```python
from build123d import *

# Parameters (mm, degrees)
SKETCH1_R           = 1.625
BOSS_EXTRUDE1_DEPTH = 2.5
FILLET1_R           = 5
SKETCH3_R           = 4.125
CUT_EXTRUDE2_DEPTH  = 71.75485849
CUT_EXTRUDE3_DEPTH  = 71.75485849
FILLET2_R           = 10
CHAMFER1_SIZE       = 1


with BuildPart() as part:
    # Sketch1 → Boss-Extrude1 (new body)
    with BuildSketch(Plane(origin=(0, 0, 0), x_dir=(1, 0, 0), z_dir=(0, 1, 0))):
        with BuildLine():
            ThreePointArc((50, 0), (-27.838821814, 41.533119315), (-19, -46.249324319))
            Line((-19, -46.249324319), (-19, -11))
            Line((-19, -11), (19, -11))
            Line((19, -11), (19, -46.249324319))
            ThreePointArc((19, -46.249324319), (41.533119315, -27.838821814), (50, 0))
        make_face()
        with Locations(Location((-15, 5, 0), (0, 0, 270))):
            Circle(SKETCH1_R, mode=Mode.SUBTRACT)
        with Locations(Location((15, 5, 0), (0, 0, 270))):
            Circle(SKETCH1_R, mode=Mode.SUBTRACT)
    extrude(amount=BOSS_EXTRUDE1_DEPTH)

    # Fillet1
    fillet1_edges = [part.edges().sort_by_distance(p)[0] for p in [
        (19, 1.25, 46.249324319),
        (19, 1.25, 11),
        (-19, 1.25, 11),
        (-19, 1.25, 46.249324319),
    ]]
    fillet(fillet1_edges, radius=FILLET1_R)

    # Sketch3 → Cut-Extrude2 (cut, through all)
    with BuildSketch(Plane(origin=(0, 2.5, 0), x_dir=(1, 0, 0), z_dir=(0, 1, 0))):
        with Locations(Location((0, 33.5, 0), (0, 0, 270))):
            Circle(SKETCH3_R)
        with Locations(Location((29.011851027, -16.75, 0), (0, 0, 270))):
            Circle(SKETCH3_R)
        with Locations(Location((-29.011851027, -16.75, 0), (0, 0, 270))):
            Circle(SKETCH3_R)
    extrude(amount=-CUT_EXTRUDE2_DEPTH, mode=Mode.SUBTRACT)

    # Sketch4 → Cut-Extrude3 (cut, through all)
    with BuildSketch(Plane(origin=(0, 2.5, 0), x_dir=(1, 0, 0), z_dir=(0, 1, 0))):
        with BuildLine():
            ThreePointArc((-19, -30.369481935), (-30.236455629, -33.609056698), (-40.88679997, -28.779673178))
            ThreePointArc((-40.88679997, -28.779673178), (-34.446124239, -36.241751129), (-26.666666667, -42.295258468))
            ThreePointArc((-26.666666667, -42.295258468), (-21.584770542, -42.4437078), (-19, -38.065732621))
            Line((-19, -38.065732621), (-19, -30.369481935))
        make_face()
        with BuildLine():
            Line((19, -30.369481935), (19, -38.065732621))
            ThreePointArc((19, -38.065732621), (21.584770542, -42.4437078), (26.666666667, -42.295258468))
            ThreePointArc((26.666666667, -42.295258468), (34.446124239, -36.241751129), (40.88679997, -28.779673178))
            ThreePointArc((40.88679997, -28.779673178), (30.236455629, -33.609056698), (19, -30.369481935))
        make_face()
        with BuildLine():
            ThreePointArc((-6.8e-08, 50), (-42.136436408, 26.916922685), (-45.36732807, -21.019170864))
            ThreePointArc((-45.36732807, -21.019170864), (-44.746417351, -10.573360804), (-38.095485584, -2.49464899))
            Line((-38.095485584, -2.49464899), (-20.59178284, 8.658863751))
            Line((-20.59178284, 8.658863751), (-16.301275801, 36.053117163))
            ThreePointArc((-16.301275801, 36.053117163), (-10.7266856, 46.037472474), (-6.8e-08, 50))
        make_face()
        with BuildLine():
            ThreePointArc((45.36732807, -21.019170864), (42.136436371, 26.916922743), (-6.8e-08, 50))
            ThreePointArc((-6.8e-08, 50), (10.726685548, 46.037472518), (16.301275801, 36.053117163))
            Line((16.301275801, 36.053117163), (20.59178284, 8.658863751))
            Line((20.59178284, 8.658863751), (38.095485584, -2.49464899))
            ThreePointArc((38.095485584, -2.49464899), (44.746417351, -10.573360804), (45.36732807, -21.019170864))
        make_face()
    extrude(amount=-CUT_EXTRUDE3_DEPTH, mode=Mode.SUBTRACT)

    # Fillet2
    fillet2_edges = [part.edges().sort_by_distance(p)[0] for p in [
        (40.88679997, 1.25, 28.779673178),
        (-45.36732807, 1.25, 21.019170864),
        (-20.59178284, 1.25, -8.658863751),
        (45.36732807, 1.25, 21.019170864),
        (20.59178284, 1.25, -8.658863751),
        (-40.88679997, 1.25, 28.779673178),
        (-19, 1.25, 30.369481935),
        (19, 1.25, 30.369481935),
    ]]
    fillet(fillet2_edges, radius=FILLET2_R)

    # Chamfer1
    chamfer1_edges = [part.edges().sort_by_distance(p)[0] for p in [
        (-44.388404549, 2.5, 9.729383862),
        (-18.097260259, 2.5, -24.5860218),
        (-44.388404549, 0, 9.729383862),
        (-18.097260259, 0, -24.5860218),
        (-43.301270189, 2.5, 25),
        (-43.301270189, 0, 25),
        (-34.559008869, 2.5, 32.717356984),
        (-19, 2.5, 19.826732149),
        (34.559008869, 2.5, 32.717356984),
        (43.301270189, 2.5, 25),
        (44.388404549, 2.5, 9.729383862),
        (31.247232254, 2.5, -1.86911803),
        (-31.247232254, 2.5, -1.86911803),
        (21.922865426, 2.5, 30.718460138),
        (-21.922865426, 2.5, 30.718460138),
        (40.660570606, 2.5, 28.929698969),
        (45.384139534, 2.5, 20.748237593),
        (-45.384139534, 2.5, 20.748237593),
        (-40.660570606, 2.5, 28.929698969),
        (-34.559008869, 0, 32.717356984),
        (-31.247232254, 0, -1.86911803),
        (31.247232254, 0, -1.86911803),
        (44.388404549, 0, 9.729383862),
        (43.301270189, 0, 25),
        (34.559008869, 0, 32.717356984),
        (-19, 0, 19.826732149),
        (21.922865426, 0, 30.718460138),
        (-21.922865426, 0, 30.718460138),
        (40.660570606, 0, 28.929698969),
        (45.384139534, 0, 20.748237593),
        (-45.384139534, 0, 20.748237593),
        (-40.660570606, 0, 28.929698969),
        (21.40495945, 2.5, -9.190948509),
        (21.40495945, 0, -9.190948509),
        (-21.40495945, 2.5, -9.190948509),
        (-21.40495945, 0, -9.190948509),
        (19, 0, 19.826732149),
        (0, 0, 11),
        (19, 2.5, 19.826732149),
        (0, 2.5, 11),
        (17.535533906, 0, 12.464466094),
        (17.535533906, 2.5, 12.464466094),
        (-17.535533906, 0, 12.464466094),
        (-17.535533906, 2.5, 12.464466094),
        (18.097260259, 0, -24.5860218),
        (0, 2.5, -50),
        (0, 0, -50),
        (18.097260259, 2.5, -24.5860218),
    ]]
    chamfer(chamfer1_edges, length=CHAMFER1_SIZE)


solid = part.part
```
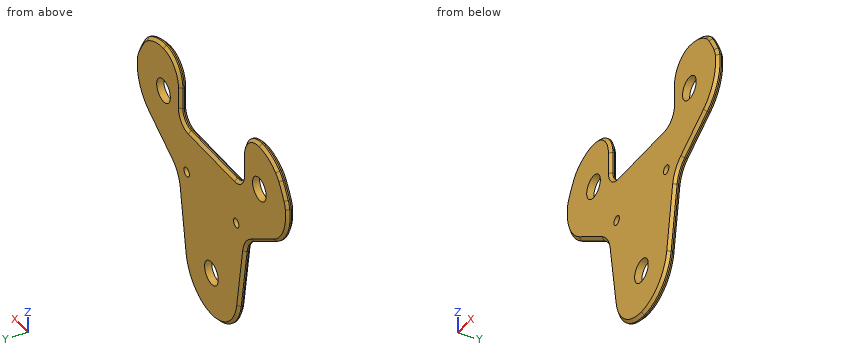
Model file for the job. Use its own axes, mm. Coordinates: 2 decimals unless noted, no trailing zeros. Order: outer loops, then holes, each group sorted by start corner. A loop starts at its lowest first (then second) coordinate and runs counter-clockwise, first axis right, second up. Notation, with made-up numbers: (35, -33.5) -> (49, -33.5) arc R19 cw to (49, -8.5) -> close; hole circle Ø7 at (-30, 9). An arc over 180 degrees is marked (long way). Answer as a JSON object with one key per item and string values. Group by question number.
1) Flat gauge pins, fed straight in: pin 1 (1.9 mm diameter, centred on x = -15, z = -5, fed in from -Y); pin 2 (1 mm diameter, centred on y = 1.5, z = -19, fed in from -X); pin 3 (1 mm diameter, centred on y = 1, z = 14, fed in from +X); pin 4 (0.6 mm diameter, centred on x = 5, y = 1.5, fed in from +Z). Where does each tip first touch, or does it go through?
2) Cut at A-A, the plane z = -33.5. Write the cut outline in (x, y) (3 decimals), then the cut area to 3 significant figures.
3) Drill centre lines: L1, parallel to X at y = 1.25, z = 16.75; L2, parallel to X at y = 1.4, z = -5 (3 decimals); L3, parallel to X at y = 1.6, z = 15. Where is each one in solid material? Low to high.
Check values:
{
 "1": {"pin 1": "passes through", "pin 2": "stops at x = -19.05", "pin 3": "stops at x = 45.76", "pin 4": "stops at z = 11"},
 "2": {"outline": "(-16.701, 1) -> (-15.689, 0) -> (-4.125, 0) -> (-4.125, 2.5) -> (-15.689, 2.5) -> (-16.701, 1.5) -> close; (4.125, 0) -> (15.689, 0) -> (16.701, 1) -> (16.701, 1.5) -> (15.689, 2.5) -> (4.125, 2.5) -> close", "area": "60.9 mm²"},
 "3": {"L1": "x = -45.92 to -33.14, -24.89 to -19, 19 to 24.89, 33.14 to 45.92", "L2": "x = -26.334 to -16.625, -13.375 to 13.375, 16.625 to 26.334", "L3": "x = -45.72 to -32.75, -25.28 to -19, 19 to 25.28, 32.75 to 45.72"}
}
